from build123d import *

# Parameters (mm, degrees)
SKETCH1_W               = 8
SKETCH1_H               = 8
BOSS_EXTRUDE1_DEPTH     = 3
CUT_EXTRUDE1_DEPTH      = 12.704699911
CUT_EXTRUDE1_DEPTH_BACK = 12.704699911
CUT_EXTRUDE2_DEPTH      = 11
SKETCH4_R               = 1.75
CUT_EXTRUDE3_DEPTH      = 0.4
SKETCH5_W               = 8
SKETCH5_H               = 1
BOSS_EXTRUDE2_DEPTH     = 2
FILLET1_R               = 4
CUT_EXTRUDE4_DEPTH      = 0.4
CUT_EXTRUDE5_DEPTH      = 0.5


with BuildPart() as part:
    # Sketch1 → Boss-Extrude1 (new body)
    with BuildSketch(Plane(origin=(0, 0, 0), x_dir=(1, 0, 0), z_dir=(0, 1, 0))):
        with Locations((4, 4)):
            Rectangle(SKETCH1_W, SKETCH1_H)
    extrude(amount=BOSS_EXTRUDE1_DEPTH)

    # Sketch2 → Cut-Extrude1 (cut, two sides: drawn at the far end of the back side and taken through both)
    with BuildSketch(Plane.XY.offset(-CUT_EXTRUDE1_DEPTH_BACK)):
        Polygon((0, 0), (0.6, 3), (0, 3), align=None)
        Polygon((8, 0), (7.4, 3), (8, 3), align=None)
    extrude(amount=CUT_EXTRUDE1_DEPTH + CUT_EXTRUDE1_DEPTH_BACK, mode=Mode.SUBTRACT)

    # Sketch3 → Cut-Extrude2 (cut)
    with BuildSketch(Plane(origin=(0, 0, 0), x_dir=(0, 0, -1), z_dir=(1, 0, 0))):
        Polygon((0, 0), (0.6, 3), (0, 3), align=None)
        Polygon((8, 3), (7.4, 3), (8, 0), align=None)
    extrude(amount=CUT_EXTRUDE2_DEPTH, mode=Mode.SUBTRACT)

    # Sketch4 → Cut-Extrude3 (cut)
    with BuildSketch(Plane.XZ):
        with Locations(Location((4, -3.75, 0), (0, 0, 270))):
            Circle(SKETCH4_R)
    extrude(amount=-CUT_EXTRUDE3_DEPTH, mode=Mode.SUBTRACT)

    # Sketch5 → Boss-Extrude2 (add)
    with BuildSketch(Plane.XZ):
        with Locations((4, -7.5)):
            Rectangle(SKETCH5_W, SKETCH5_H)
    extrude(amount=BOSS_EXTRUDE2_DEPTH)

    # Fillet1
    # the kernel refuses this fillet: 4 mm, written as the material it takes off along each edge
    with BuildSketch(Plane(origin=(8, -2, -16.660254038), x_dir=(0, 1, 0), z_dir=(0, 0, 1)), Plane(origin=(0, -2, 1.660254038), x_dir=(0, 1, 0), z_dir=(0, 0, -1))) as fillet1_piece_1:
        with BuildLine():
            CenterArc((4, 3.464101615), FILLET1_R, 180, 60)
            Line((0, 3.464101615), (-0.08, 3.464101615))
            Line((-0.08, 3.464101615), (-0.08, 0))
            Line((-0.08, 0), (0, -0.08))
            ThreePointArc((0, -0.08), (1, -0.08), (1.96, -0.069282032))
            Line((1.96, -0.069282032), (2, 0))
        make_face()
    extrude(amount=18.320508076, mode=Mode.SUBTRACT)

    # Sketch6 → Cut-Extrude4 (cut)
    with BuildSketch(Plane(origin=(0, 3, 0), x_dir=(1, 0, 0), z_dir=(0, 1, 0))):
        Polygon((3.652362984, 2.002856352), (3.652362984, 5.336189685), (2.472875805, 5.336189685), (2.472875805, 6.002856352), (5.601080933, 6.002856352), (5.601080933, 5.336189685), (4.421593754, 5.336189685), (4.421593754, 2.002856352), align=None)
    extrude(amount=-CUT_EXTRUDE4_DEPTH, mode=Mode.SUBTRACT)

    # Sketch7 → Cut-Extrude5 (cut)
    with BuildSketch(Plane(origin=(0, 3, 0), x_dir=(1, 0, 0), z_dir=(0, 1, 0))):
        with BuildLine():
            Line((5.873519392, 1.453659702), (6.173519392, 1.492602009))
            add(Edge.make_bspline(
                [(6.173519392, 1.492602009), (6.1768382, 1.472256976), (6.18322911, 1.433079261), (6.203068429, 1.378384162), (6.230697403, 1.330199963), (6.266205672, 1.289626965), (6.30661854, 1.256629271), (6.351264588, 1.233104776), (6.398791495, 1.218293755), (6.431707248, 1.216554551), (6.448279008, 1.215678932)],
                knots=[0, 0, 0, 0, 1.154848647, 2.223851388, 3.245409892, 4.254330626, 5.232966172, 6.156270698, 7.071756339, 8, 8, 8, 8], degree=3))
            add(Edge.make_bspline(
                [(6.448279008, 1.215678932), (6.457906388, 1.215848075), (6.476752132, 1.216179174), (6.504524052, 1.219937575), (6.531053869, 1.226043662), (6.55659259, 1.234330756), (6.580874213, 1.245230043), (6.603920328, 1.258567919), (6.625817059, 1.274363121), (6.646675237, 1.292223374), (6.665948362, 1.312615024), (6.682055884, 1.336087325), (6.696325112, 1.361440746), (6.707949377, 1.389364059), (6.716328852, 1.41995512), (6.722995329, 1.45269023), (6.726393576, 1.487964606), (6.7270346, 1.51218758), (6.727365546, 1.524693355)],
                knots=[0, 0, 0, 0, 0.981268084, 1.920847364, 2.851509818, 3.754644372, 4.654445699, 5.560569672, 6.465366234, 7.403985617, 8.358004942, 9.316972086, 10.299158387, 11.321223707, 12.392031981, 13.529051644, 14.724304971, 16, 16, 16, 16], degree=3))
            add(Edge.make_bspline(
                [(6.727365546, 1.524693355), (6.727178419, 1.536481523), (6.726816764, 1.559264099), (6.723461454, 1.592272205), (6.718311073, 1.623118586), (6.710117629, 1.651577708), (6.700760071, 1.678178631), (6.688143723, 1.701978526), (6.674300374, 1.724011312), (6.657427434, 1.743088207), (6.639042824, 1.759943867), (6.619463278, 1.774961982), (6.598469004, 1.787493154), (6.576269045, 1.79824857), (6.552478567, 1.806082762), (6.527290541, 1.811294815), (6.501043648, 1.815207497), (6.483029864, 1.815520133), (6.473879969, 1.815678932)],
                knots=[0, 0, 0, 0, 1.29221626, 2.497420946, 3.635005972, 4.715822244, 5.741640361, 6.720139245, 7.663294346, 8.588224307, 9.502291809, 10.395891443, 11.288713187, 12.178904539, 13.095818132, 14.026458458, 14.997562253, 16, 16, 16, 16], degree=3))
            add(Edge.make_bspline(
                [(6.473879969, 1.815678932), (6.462311673, 1.815264192), (6.439232742, 1.814436778), (6.405164091, 1.807710713), (6.372003678, 1.796760631), (6.339785969, 1.781517356), (6.308596201, 1.761859078), (6.278569411, 1.737720606), (6.249190173, 1.70951724), (6.23114374, 1.688207441), (6.2218367, 1.677217394)],
                knots=[0, 0, 0, 0, 0.931687088, 1.85873035, 2.786835662, 3.740075265, 4.723687035, 5.750832598, 6.840042753, 8, 8, 8, 8], degree=3))
            Line((6.2218367, 1.677217394), (5.919673238, 1.719765471))
            Line((5.919673238, 1.719765471), (6.127365546, 2.715678932))
            Line((6.127365546, 2.715678932), (7.004288623, 2.715678932))
            Line((7.004288623, 2.715678932), (7.004288623, 2.369525086))
            Line((7.004288623, 2.369525086), (6.405009777, 2.369525086))
            Line((6.405009777, 2.369525086), (6.3343367, 2.048251048))
            add(Edge.make_bspline(
                [(6.3343367, 2.048251048), (6.352346227, 2.058641979), (6.3874181, 2.078877348), (6.443410579, 2.099707804), (6.499690691, 2.113077126), (6.537629531, 2.114816152), (6.556452085, 2.115678932)],
                knots=[0, 0, 0, 0, 1.060051984, 2.064352337, 3.039669322, 4, 4, 4, 4], degree=3))
            add(Edge.make_bspline(
                [(6.556452085, 2.115678932), (6.574146885, 2.115202759), (6.60910097, 2.114262131), (6.660364054, 2.106544582), (6.709535097, 2.093825268), (6.756780138, 2.076125011), (6.801761249, 2.052924592), (6.844866196, 2.024883357), (6.885472675, 1.991514713), (6.924016987, 1.953782044), (6.959166694, 1.912035385), (6.989521263, 1.866512768), (7.015738821, 1.818347997), (7.037083021, 1.767008911), (7.053155816, 1.712424088), (7.065192785, 1.655063547), (7.07193581, 1.594565079), (7.072984339, 1.553314949), (7.073519392, 1.532265471)],
                knots=[0, 0, 0, 0, 0.974409932, 1.924837087, 2.848242317, 3.768103797, 4.697919751, 5.630842317, 6.595644344, 7.588240789, 8.59876155, 9.595918743, 10.597287627, 11.615415169, 12.652315553, 13.727511434, 14.840374562, 16, 16, 16, 16], degree=3))
            add(Edge.make_bspline(
                [(7.073519392, 1.532265471), (7.073036469, 1.514585649), (7.072077961, 1.479494734), (7.066471429, 1.42756738), (7.056005109, 1.377169317), (7.042672536, 1.328016631), (7.024246745, 1.280521142), (7.002381003, 1.234373213), (6.976242653, 1.189655711), (6.956076521, 1.161441782), (6.945875162, 1.147169317)],
                knots=[0, 0, 0, 0, 1.027524957, 2.039431707, 3.02972907, 4.015954419, 4.995255842, 5.985553205, 6.980960039, 8, 8, 8, 8], degree=3))
            add(Edge.make_bspline(
                [(6.945875162, 1.147169317), (6.931003624, 1.128791302), (6.901734709, 1.092621232), (6.851630217, 1.045066578), (6.797135444, 1.00512898), (6.738397987, 0.97233011), (6.675480422, 0.946591981), (6.608098871, 0.928697649), (6.536747385, 0.917626673), (6.487743367, 0.916337636), (6.462702085, 0.915678932)],
                knots=[0, 0, 0, 0, 1.018121711, 2.003781959, 2.967346956, 3.92281574, 4.896313303, 5.889026666, 6.921282725, 8, 8, 8, 8], degree=3))
            add(Edge.make_bspline(
                [(6.462702085, 0.915678932), (6.442489279, 0.916044029), (6.403022672, 0.9167569), (6.345224712, 0.92380666), (6.290451314, 0.935259909), (6.238356922, 0.95115359), (6.18925085, 0.971795666), (6.142751555, 0.99671717), (6.099246456, 1.026470486), (6.058935891, 1.060830838), (6.021919655, 1.09880899), (5.988902802, 1.140363971), (5.959526451, 1.184800784), (5.934351052, 1.232568443), (5.912895663, 1.28333195), (5.895811978, 1.337351468), (5.881746134, 1.394266746), (5.876291993, 1.433642912), (5.873519392, 1.453659702)],
                knots=[0, 0, 0, 0, 1.098912142, 2.145685936, 3.161086862, 4.139124218, 5.10307886, 6.053641493, 7.003731987, 7.963777669, 8.929946266, 9.883471279, 10.846206077, 11.822909928, 12.81603559, 13.839338588, 14.901632394, 16, 16, 16, 16], degree=3))
        make_face()
    extrude(amount=-CUT_EXTRUDE5_DEPTH, mode=Mode.SUBTRACT)


solid = part.part
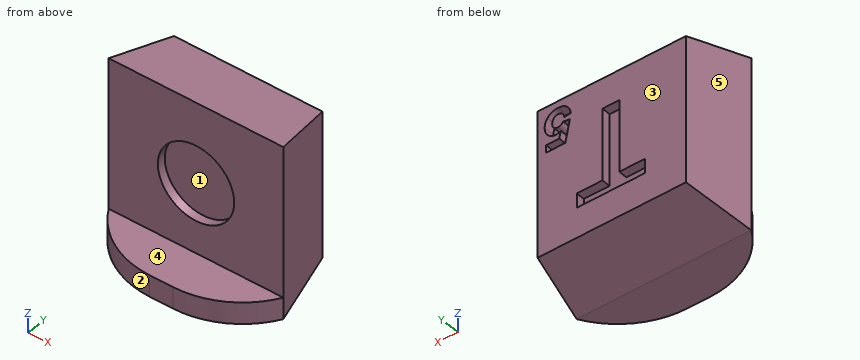
The model under review builds one solid part; all positions refer to its coordinate system, in mm. Face numbers are marked on the shaded views. A direction names the side the tool comes from. Coordinates: 2 decimals unless noted, no trailing zeros. Loops run counter-clockwise (first coordinate to the right, second up) from the corner with the lowest first, then second, coordinate; pieces in that order, holes last.
(1) Insertion check: P1, Ø0.6, axis at x = 3.5, y = -1, coming from the +Z side; P2, Ø4, axis at x = 4, z = -3.75, coming from the -Y side. Each pin has a flat end and moves straight along its axis. Give the tip position at first contact, or say it passes through.
Determined:
P1: stops at z = -7
P2: stops at y = 0
(2) Draft analysis for pull direction X (two halves, no side actions). For the marked faces 1, 2 and 3, state which applies: +X half, -X half, draft (parallel to the pull), parting line (faces both ways), or undercut.
Determined:
face 1: undercut
face 2: -X half
face 3: draft
(3) Consider section D-D, the plane x = 1.75. Give the boundary of the cut face in (y, z), plus the area to 3 significant figures.
Determined:
outline: (-1.61, -8) - (0, -8) - (3, -7.4) - (3, -0.6) - (0, 0) - (0, -7) - (-1.61, -7) - close
area: 23.8 mm2
(4) Consider section B-B, the plane z = -3.75. Give the boundary of the cut face in (x, y).
Determined:
outline: (0, 0) - (2.25, 0) - (2.25, 0.4) - (5.75, 0.4) - (5.75, 0) - (8, 0) - (7.4, 3) - (4.42, 3) - (4.42, 2.6) - (3.65, 2.6) - (3.65, 3) - (0.6, 3) - close
(5) Wall thickness on L1, parallel to Y at x = 4, z = -2.5; L2, parallel to Y at x = 3.25, z = -6.5; L3, parallel to Z at x = 0.5, y = -0.05: over which ranges is each line inside the solid? List them lowest first.
Determined:
L1: y = 0.4 to 2.6
L2: y = 0 to 3
L3: z = -8 to -7
(6) Tool access review of the marked faces 4 and 5: name each direction out of +Z, -Z, +X, -X, +Y, -Y from which nothing blocks a thin tool from reaching the whole face with its end or side.
Determined:
face 4: +Z, +X, -X, -Y
face 5: +Z, -Z, -X, +Y
(7) Consider section C-C, the plane y = 0.55. Give the boundary of the cut face in (x, z).
Determined:
outline: (0.11, -7.89) - (7.89, -7.89) - (7.89, -0.11) - (0.11, -0.11) - close
(8) Consider section A-A, the plane x = 4. Give the boundary of the cut face in (y, z), plus the area to 3 significant figures.
Determined:
outline: (-2, -8) - (0, -8) - (3, -7.4) - (3, -6) - (2.6, -6) - (2.6, -2) - (3, -2) - (3, -0.6) - (0, 0) - (0, -2) - (0.4, -2) - (0.4, -5.5) - (0, -5.5) - (0, -7) - (-2, -7) - close
area: 21.2 mm2
